Source: CAD feature listing. Evaluate the final solid. Frame: model axes, mm. A direction names the side the tool comes from. Round coordinates to 2 decimals unless told otherwise and drop trailing zeros. Loops run counter-clockwise (first coordinate to the right, second up) from the corner with the lowest first, then second, coordinate; pieces in that order, holes last.
(1) Section D-D, the plane x = 2.25. Return the cut outline in (y, z), plus the area to 3 significant figures.
(2) Mould query, pull axis Y, two halves, no side actions, for faces 1 (the cylindrical face through (4.972, -8.738, -0.493)), 2 (the cylindrical face through (-0.1, 8.5, -0.5)), 3 (the cylindrical face through (-5.188, -8.738, -0.493)), 4 (the cylindrical face through (-8.33, -1.69, -0.49)). Classes: pulls with the +Y half, pulls with the -Y half, needs draft (parallel to the pull), parting line crosses it, or undercut.
(3) Section A-A, the plane y = -8.25. Return the cut outline in (x, z), plus the area to 3 significant figures.
(4) Section B-B, the plane x = 0. Return the cut outline in (y, z), plus the area to 3 significant figures.
(5) Material intervals for probe 1 along X at (y, z) = (0, -0.1); probe 2 along X at (y, z) = (1, -0.2); probe 3 along X at (y, z) = (-9.5, -0.6), sorted ascending.
(6) First-contact query: pin 1 Ø0.5 at (y, z) = (-11, -0.5) entering from -X; pin 2 Ø0.6 at (x, z) = (8, -0.5) entering from -Y; pin 3 Ø5 at (x, y) = (0, 0) entering from +Z. Flat tips, straight axial feed; report the tip coordinate or a pass-through.
(7) Section C-C, the plane y = 2.5. Return the cut outline in (x, z), plus the area to 3 significant figures.
(8) Set-up query: faces 5 (the flat face through (8.1, -0.4, -0.5)), 6 (the flat face through (-8.1, 0.4, -0.5)), 7 (the flat face through (-6.963, -8.1, -0.5)), 8 (the flat face through (0, -10.5, -0.5)). Return all of +Z, -Z, +X, -X, +Y, -Y with unobstructed straight access to the full face (end or side cutting, diameter ignored); none if empty.
```python
from build123d import *

# Parameters (mm, degrees)
SKETCH006_R     = 3
PAD005_DEPTH    = 1
SKETCH016_R     = 0.5
POCKET004_DEPTH = 2
POCKET005_DEPTH = 5


with BuildPart() as part:
    # Sketch006 (on ShapeBinder) → Pad005 (new body)
    with BuildSketch(Plane(origin=(0, 0, 0), x_dir=(1, 0, 0), z_dir=(0, 0, -1))):
        with BuildLine():
            ThreePointArc((-7.987387, 2.907171), (-8.333808, 1.672617), (-8.490583, 0.4))
            Line((-7.689603, 0.4), (-8.490583, 0.4))
            ThreePointArc((-7.689603, 0.4), (-7.7, 0), (-7.689603, -0.4))
            Line((-7.689603, -0.4), (-8.490583, -0.4))
            ThreePointArc((-8.490583, -0.4), (-8.333808, -1.672617), (-7.987387, -2.907171))
            Line((-7.987387, -2.907171), (-7.496671, -2.792834))
            ThreePointArc((-7.496671, -2.792834), (-7.082093, -3.720747), (-6.553216, -4.588611))
            Line((-6.962792, -4.8754), (-6.553216, -4.588611))
            ThreePointArc((-6.962792, -4.8754), (0, -8.5), (6.962792, -4.8754))
            Line((6.962792, -4.8754), (6.553216, -4.588611))
            ThreePointArc((6.553216, -4.588611), (7.082093, -3.720747), (7.496671, -2.792834))
            Line((7.987387, -2.907171), (7.496671, -2.792834))
            ThreePointArc((7.987387, -2.907171), (8.333808, -1.672617), (8.490583, -0.4))
            Line((8.490583, -0.4), (7.689603, -0.4))
            ThreePointArc((7.689603, -0.4), (7.7, 0), (7.689603, 0.4))
            Line((8.490583, 0.4), (7.689603, 0.4))
            ThreePointArc((8.490583, 0.4), (8.333808, 1.672617), (7.987387, 2.907171))
            Line((7.987387, 2.907171), (7.496671, 2.792834))
            ThreePointArc((7.496671, 2.792834), (7.082093, 3.720747), (6.553216, 4.588611))
            Line((6.962792, 4.8754), (6.553216, 4.588611))
            Line((6.962792, 4.8754), (6.962792, 11.5))
            Line((6.962792, 11.5), (-6.962792, 11.5))
            Line((-6.962792, 4.8754), (-6.962792, 11.5))
            Line((-6.962792, 4.8754), (-6.553216, 4.588611))
            ThreePointArc((-6.553216, 4.588611), (-7.082093, 3.720747), (-7.496671, 2.792834))
            Line((-7.987387, 2.907171), (-7.496671, 2.792834))
        make_face()
        Circle(SKETCH006_R, mode=Mode.SUBTRACT)
    extrude(amount=PAD005_DEPTH)

    # Sketch016 (on Face28 of Pad005) → Pocket004 (cut)
    with BuildSketch(Plane.XY):
        with Locations((0, -8.25)):
            Circle(SKETCH016_R)
        with Locations((-5.08, -8.25)):
            Circle(SKETCH016_R)
        with Locations((5.08, -8.25)):
            Circle(SKETCH016_R)
    extrude(amount=-POCKET004_DEPTH, mode=Mode.SUBTRACT)

    # Sketch017 (on Face4 of Pocket004) → Pocket005 (cut)
    with BuildSketch(Plane.XY):
        Polygon((-6.962792, -11.5), (-6, -11.5), (-6, -10.5), (-4.5, -10.5), (-4.5, -11.5), (-0.75, -11.5), (-0.75, -10.5), (0.75, -10.5), (0.75, -11.5), (4.33, -11.5), (4.33, -10.5), (5.83, -10.5), (5.83, -11.5), (6.962792, -11.5), (6.962792, -12.871278), (-6.962792, -12.871278), align=None)
    extrude(amount=-POCKET005_DEPTH, mode=Mode.SUBTRACT)


solid = part.part
```
Output values:
1. outline: (-11.5, -1) - (-1.98, -1) - (-1.98, 0) - (-11.5, 0) - close; (1.98, -1) - (8.2, -1) - (8.2, 0) - (1.98, 0) - close
1. area: 15.7 mm2
2. face 1: undercut
2. face 2: pulls with the +Y half
2. face 3: undercut
2. face 4: pulls with the -Y half
3. outline: (-6.96, -1) - (-5.58, -1) - (-5.58, 0) - (-6.96, 0) - close; (-4.58, -1) - (-0.5, -1) - (-0.5, 0) - (-4.58, 0) - close; (0.5, -1) - (4.58, -1) - (4.58, 0) - (0.5, 0) - close; (5.58, -1) - (6.96, -1) - (6.96, 0) - (5.58, 0) - close
3. area: 10.9 mm2
4. outline: (-10.5, -1) - (-8.75, -1) - (-8.75, 0) - (-10.5, 0) - close; (-7.75, -1) - (-3, -1) - (-3, 0) - (-7.75, 0) - close; (3, -1) - (8.5, -1) - (8.5, 0) - (3, 0) - close
4. area: 12.0 mm2
5. probe 1: x = -7.7 to -3, 3 to 7.7
5. probe 2: x = -8.44 to -2.83, 2.83 to 8.44
5. probe 3: x = -6.96 to 6.96
6. pin 1: stops at x = -6.96
6. pin 2: stops at y = -2.91
6. pin 3: passes through
7. outline: (-8.12, -1) - (-1.66, -1) - (-1.66, 0) - (-8.12, 0) - close; (1.66, -1) - (8.12, -1) - (8.12, 0) - (1.66, 0) - close
7. area: 12.9 mm2
8. face 5: +Z, -Z, +X
8. face 6: +Z, -Z, -X
8. face 7: +Z, -Z, -X, -Y
8. face 8: +Z, -Z, -Y
